```python
from build123d import *

# Parameters (mm, degrees)
SKETCH3_W                = 55
SKETCH3_H                = 77.5
SKETCH3_R                = 20
SKETCH3_R_2              = 1.6
BOSS_EXTRUDE1_DEPTH      = 3
SKETCH4_W                = 55
SKETCH4_H                = 77.5
SKETCH4_R                = 25
BOSS_EXTRUDE2_DEPTH      = 10
SKETCH5_R                = 4
CUT_EXTRUDE1_DEPTH       = 11
FILLET1_R                = 3
FILLET2_R                = 6
SKETCH6_W                = 55
SKETCH6_H                = 18
BOSS_EXTRUDE3_DEPTH      = 10
SKETCH7_R                = 4.4323
TRIPODMOUNT_DEPTH        = 12
FILLET3_R                = 3
CHAMFER1_SIZE            = 0.5
CHAMFER3_SIZE            = 0.5
CHAMFERTRIPODMOUNT_SIZE  = 0.3048
CHAMFERTRIPODMOUNT_SIZE2 = 4.358843075


with BuildPart() as part:
    # Sketch3 → Boss-Extrude1 (new body)
    with BuildSketch(Plane(origin=(0, 0, 0), x_dir=(1, 0, 0), z_dir=(0, 1, 0))):
        with Locations((0, -11.25)):
            Rectangle(SKETCH3_W, SKETCH3_H)
        with Locations(Location((0, 0, 0), (0, 0, 270))):  # turned: the seam where the file's is
            Circle(SKETCH3_R, mode=Mode.SUBTRACT)
        with Locations(Location((-20, 20, 0), (0, 0, 270))):  # turned: the seam where the file's is
            Circle(SKETCH3_R_2, mode=Mode.SUBTRACT)
        with Locations(Location((20, 20, 0), (0, 0, 270))):  # turned: the seam where the file's is
            Circle(SKETCH3_R_2, mode=Mode.SUBTRACT)
        with Locations(Location((20, -20, 0), (0, 0, 270))):  # turned: the seam where the file's is
            Circle(SKETCH3_R_2, mode=Mode.SUBTRACT)
        with Locations(Location((-20, -20, 0), (0, 0, 270))):  # turned: the seam where the file's is
            Circle(SKETCH3_R_2, mode=Mode.SUBTRACT)
    extrude(amount=BOSS_EXTRUDE1_DEPTH)

    # Sketch4 → Boss-Extrude2 (add)
    with BuildSketch(Plane(origin=(0, 3, 0), x_dir=(1, 0, 0), z_dir=(0, 1, 0))):
        with Locations((0, -11.25)):
            Rectangle(SKETCH4_W, SKETCH4_H)
        with Locations(Location((0, 0, 0), (0, 0, 270))):  # turned: the seam where the file's is
            Circle(SKETCH4_R, mode=Mode.SUBTRACT)
    extrude(amount=BOSS_EXTRUDE2_DEPTH)

    # Sketch5 → Cut-Extrude1 (cut, through all)
    with BuildSketch(Plane.XZ.offset(-3)):
        with Locations((20, -20)):
            Circle(SKETCH5_R)
        with Locations((-20, -20)):
            Circle(SKETCH5_R)
        with Locations((-20, 20)):
            Circle(SKETCH5_R)
        with Locations((20, 20)):
            Circle(SKETCH5_R)
    extrude(amount=-CUT_EXTRUDE1_DEPTH, mode=Mode.SUBTRACT)

    # Fillet1
    fillet1_edges = [part.edges().sort_by_distance(p)[0] for p in [
        (16.095976426, 8, 19.129023574),
        (19.129023574, 8, 16.095976426),
        (-19.129023574, 8, 16.095976426),
        (-16.095976426, 8, 19.129023574),
        (-16.095976426, 8, -19.129023574),
        (-19.129023574, 8, -16.095976426),
        (19.129023574, 8, -16.095976426),
        (16.095976426, 8, -19.129023574),
    ]]
    fillet(fillet1_edges, radius=FILLET1_R)

    # Fillet2
    fillet2_edges = [part.edges().sort_by_distance(p)[0] for p in [
        (-27.5, 6.5, -27.5),
        (27.5, 6.5, -27.5),
    ]]
    fillet(fillet2_edges, radius=FILLET2_R)

    # Sketch6 → Boss-Extrude3 (add)
    with BuildSketch(Plane(origin=(0, 13, 0), x_dir=(1, 0, 0), z_dir=(0, 1, 0))):
        with Locations((0, -41)):
            Rectangle(SKETCH6_W, SKETCH6_H)
    extrude(amount=BOSS_EXTRUDE3_DEPTH)

    # Sketch7 → TripodMount (cut)
    with BuildSketch(Plane.XY.offset(50)):
        with Locations((0, 11.5)):
            Circle(SKETCH7_R)
    extrude(amount=-TRIPODMOUNT_DEPTH, mode=Mode.SUBTRACT)

    # Fillet3
    fillet3_edges = [part.edges().sort_by_distance(p)[0] for p in [
        (-27.5, 18, 32),
        (27.5, 18, 32),
        (-27.5, 23, 41),
        (0, 23, 50),
        (27.5, 23, 41),
        (0, 23, 32),
        (27.5, 11.5, 50),
        (-27.5, 11.5, 50),
    ]]
    fillet(fillet3_edges, radius=FILLET3_R)

    # Chamfer1
    chamfer1_edges = [part.edges().sort_by_distance(p)[0] for p in [
        (0, 0, -20),
        (0, 0, -27.5),
        (-27.5, 0, 12.75),
        (-25.742640687, 0, -25.742640687),
        (25.742640687, 0, -25.742640687),
        (20, 0, -21.6),
        (27.5, 0, 12.75),
        (0, 0, 50),
        (-26.621320344, 0, 49.121320344),
        (26.621320344, 0, 49.121320344),
        (20, 0, 18.4),
        (-20, 0, 18.4),
        (-20, 0, -21.6),
    ]]
    chamfer(chamfer1_edges, length=CHAMFER1_SIZE)

    # Chamfer3
    chamfer3_edges = [part.edges().sort_by_distance(p)[0] for p in [
        (22.828427125, 13, 22.828427125),
        (0, 13, 25),
        (-22.828427125, 13, 22.828427125),
        (-25, 13, 0),
        (-22.828427125, 13, -22.828427125),
        (0, 13, -25),
        (25, 13, 0),
        (-14.921579234, 13, -21.134173852),
        (-21.134173852, 13, -14.921579234),
        (-21.134173852, 13, 14.921579234),
        (14.921579234, 13, -21.134173852),
        (21.134173852, 13, 14.921579234),
        (14.921579234, 13, 21.134173852),
        (-14.921579234, 13, 21.134173852),
        (21.134173852, 13, -14.921579234),
        (0, 13, -27.5),
        (-27.5, 13, 5.25),
        (-25.742640687, 13, -25.742640687),
        (25.742640687, 13, -25.742640687),
        (27.5, 13, 5.25),
        (22.828427125, 13, -22.828427125),
    ]]
    chamfer(chamfer3_edges, length=CHAMFER3_SIZE)

    # ChamferTripodMount
    chamfertripodmount_edges = [part.edges().sort_by_distance(p)[0] for p in [
        (-4.4323, 11.5, 50),
    ]]
    chamfertripodmount_side = [part.faces().sort_by_distance(p)[0] for p in [
        (23.972624422, 10.25, 50),
    ]]
    chamfer(chamfertripodmount_edges, length=CHAMFERTRIPODMOUNT_SIZE, length2=CHAMFERTRIPODMOUNT_SIZE2, reference=chamfertripodmount_side[0])


solid = part.part
```
For this review, take the finished solid that the model builds, in its own axes (mm). A direction names the side the tool comes from. Coordinates: 2 decimals unless noted, no trailing zeros. Order: outer loops, then holes, each group sorted by start corner. A loop starts at its lowest first (then second) coordinate and runs counter-clockwise, first axis right, second up. Notation, with made-up numbers: (47.5, 1.5) - (74.5, 1.5) arc R25 ccw to (74.5, 36.5) - close; hole circle Ø8 at (60.25, -12). An arc over 180 degrees is marked (long way). Answer as a JSON object with one key per item and string values. Group by question number.
1. The part is to be moulded in two halves that separate along X. For faces 1 (the flat face through (0, 0, 28)), 2 (the flat face through (27.5, 8, 13)), 3 (the flat face through (-11, 3, -17)), say which applies: pulls with the +X half, pulls with the -X half, needs draft (parallel to the pull), parting line crosses it, or undercut.
2. We need section B-B on z = 0. State the section outline as (x, y) points, then the cut area to 3 significant figures.
3. For faces 4 (the cylindrical face through (-18.414, 1.732, -20.208)), 5 (the cylindrical face through (26.6, 16.3, 32.86)), 6 (the conical face through (-25.135, 12.635, 0.189)), list the 3-axis set-ups (+Z, -Z, +X, -X, +Y, -Y) from which the entire face can be reached by the end or side of a thin tool; tool diameter is ignored.
4. For probe 1 along X at (y, z) = (9, 20); probe 2 along X at (y, z) = (2.1, 0); probe 3 along X at (y, z) = (6.75, 23), list the stretches that pass through material, from the lowest coordinate up.
5. We need section D-D on z = 28.5. State the section outline as (x, y) points, then the cut area to 4 significant figures.
6. Clearance check with flat-ended pins moving along their axes: P1, Ø13, axis at x = 20, z = -20, coming from the +Y side; P2, Ø1.5, axis at y = 15, z = 31.5, coming from the +X side; P3, Ø2.5, axis at x = -20, z = 20, coming from the -Y side; P4, Ø4, axis at x = -20, z = -20, coming from the +Y side. State where each tip first meets the part, or that it passes through.
7. We need section C-C on y = 18. State the section outline as (x, z) points.
Final values:
{
 "1": {"face 1": "needs draft", "face 2": "pulls with the +X half", "face 3": "undercut"},
 "2": {"outline": "(-27.5, 0.5) - (-27, 0) - (-20.5, 0) - (-20, 0.5) - (-20, 3) - (-25, 3) - (-25, 12.5) - (-25.5, 13) - (-27, 13) - (-27.5, 12.5) - close; (20, 0.5) - (20.5, 0) - (27, 0) - (27.5, 0.5) - (27.5, 12.5) - (27, 13) - (25.5, 13) - (25, 12.5) - (25, 3) - (20, 3) - close", "area": "94.0 mm²"},
 "3": {"face 4": "+Y, -Y", "face 5": "-Z, +X, +Y", "face 6": "+Y"},
 "4": {"probe 1": "-27.5 to -24, 24 to 27.5", "probe 2": "-27.5 to -20, 20 to 27.5", "probe 3": "-27.5 to -22.65, -17.35 to -9.8, 9.8 to 17.35, 22.65 to 27.5"},
 "5": {"outline": "(-27.5, 0.5) - (-27, 0) - (27, 0) - (27.5, 0.5) - (27.5, 12.5) - (27, 13) - (-27, 13) - (-27.5, 12.5) - close", "area": "714.5 mm²"},
 "6": {"P1": "y = 13", "P2": "x = 25.7", "P3": "through", "P4": "y = 3"},
 "7": {"outline": "(-27.5, 35) arc R3 ccw to (-24.5, 32) - (24.5, 32) arc R3 ccw to (27.5, 35) - (27.5, 47) arc R3 ccw to (24.5, 50) - (-24.5, 50) arc R3 ccw to (-27.5, 47) - close"}
}
